from build123d import *

# Parameters (mm, degrees)
SKETCH_R        = 1.55
PAD_DEPTH       = 6.3
SKETCH001_W     = 3.4
SKETCH001_H     = 7.5
PAD001_DEPTH    = 6.3
SKETCH002_W     = 10
SKETCH002_H     = 19.4
PAD002_DEPTH    = 6
SKETCH003_R     = 1.65
POCKET_DEPTH    = 6.901
SKETCH004_R     = 1.65
POCKET001_DEPTH = 3.401
SKETCH005_R     = 2.2
POCKET002_DEPTH = 5
SKETCH006_W     = 5.6
SKETCH006_H     = 5.6
POCKET003_DEPTH = 2
SKETCH007_W     = 5.6
SKETCH007_H     = 5.6
POCKET004_DEPTH = 2
FILLET_R        = 4
CHAMFER_SIZE    = 5


with BuildPart() as part:
    # Sketch → Pad (new body)
    with BuildSketch(Plane.YZ):
        Polygon((-6.9, -4.5), (0, -4.5), (0, -19), (-15, -19), (-15, -11), (-6.9, -11), align=None)
        with Locations((-11, -15)):
            Circle(SKETCH_R, mode=Mode.SUBTRACT)
        with Locations((-4, -15)):
            Circle(SKETCH_R, mode=Mode.SUBTRACT)
    extrude(amount=PAD_DEPTH)

    # Sketch001 (on Face9 of Pad) → Pad001 (join)
    with BuildSketch(Plane(origin=(0, 0, 0), x_dir=(0, 1, 0), z_dir=(-1, 0, 0))):
        with Locations((-1.7, 8.25)):
            Rectangle(SKETCH001_W, SKETCH001_H)
    extrude(amount=PAD001_DEPTH)

    # Sketch002 (on Face11 of Pad001) → Pad002 (join)
    with BuildSketch(Plane(origin=(-6.3, 0, 0), x_dir=(0, 1, 0), z_dir=(-1, 0, 0))):
        with Locations((-5, 2.3)):
            Rectangle(SKETCH002_W, SKETCH002_H)
    extrude(amount=PAD002_DEPTH)

    # Sketch003 (on Face1 of Pad002) → Pocket (cut, through all)
    with BuildSketch(Plane(origin=(0, -6.9, 0), x_dir=(0, 0, -1), z_dir=(0, -1, 0))):
        with Locations((8.25, 3.15)):
            Circle(SKETCH003_R)
    extrude(amount=-POCKET_DEPTH, mode=Mode.SUBTRACT)

    # Sketch004 (on Face11 of Pocket) → Pocket001 (cut, through all)
    with BuildSketch(Plane(origin=(0, -3.4, 0), x_dir=(0, 0, -1), z_dir=(0, -1, 0))):
        with Locations((8.25, -3.15)):
            Circle(SKETCH004_R)
    extrude(amount=-POCKET001_DEPTH, mode=Mode.SUBTRACT)

    # Sketch005 (on Face18 of Pocket001) → Pocket002 (cut)
    with BuildSketch(Plane(origin=(0, -10, 0), x_dir=(0, 0, -1), z_dir=(0, -1, 0))):
        with Locations((-2.4, -9.3)):
            Circle(SKETCH005_R)
        with Locations((2.4, -9.3)):
            Circle(SKETCH005_R)
    extrude(amount=-POCKET002_DEPTH, mode=Mode.SUBTRACT)

    # Sketch006 (on Face3 of Pocket002) → Pocket003 (cut)
    with BuildSketch(Plane(origin=(0, 0, 0), x_dir=(0, 1, 0), z_dir=(-1, 0, 0))):
        with Locations((-4, 15)):
            Rectangle(SKETCH006_W, SKETCH006_H)
        with Locations((-11, 15)):
            Rectangle(SKETCH006_W, SKETCH006_H)
    extrude(amount=-POCKET003_DEPTH, mode=Mode.SUBTRACT)

    # Sketch007 (on Face11 of Pocket003) → Pocket004 (cut)
    with BuildSketch(Plane.ZX):
        with Locations((-8.25, 3.15)):
            Rectangle(SKETCH007_W, SKETCH007_H)
        with Locations((-8.25, -3.15)):
            Rectangle(SKETCH007_W, SKETCH007_H)
    extrude(amount=-POCKET004_DEPTH, mode=Mode.SUBTRACT)

    # Fillet
    fillet_edges = [part.edges().sort_by_distance(p)[0] for p in [
        (-12.3, -5, 7.4),
    ]]
    fillet(fillet_edges, radius=FILLET_R)

    # Chamfer
    chamfer_edges = [part.edges().sort_by_distance(p)[0] for p in [
        (-12.3, -5, -12),
    ]]
    chamfer(chamfer_edges, length=CHAMFER_SIZE)


solid = part.part
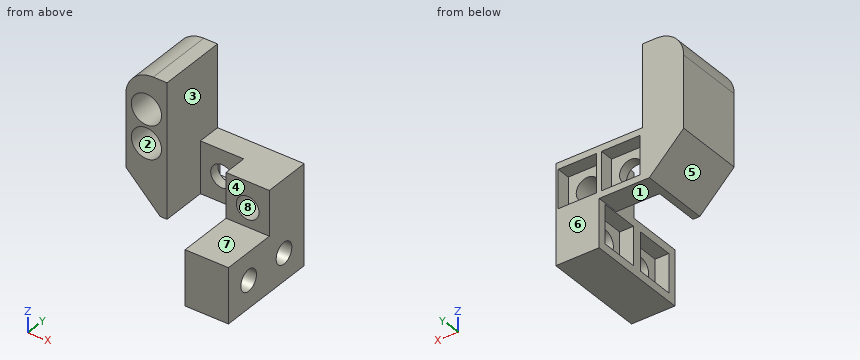
Source: CAD feature listing. Evaluate the final solid. Frame: model axes, mm. Face numbers are marked on the shaded views. A direction names the side the tool comes from. Coordinates: 2 decimals unless noted, no trailing zeros. Loops run counter-clockwise (first coordinate to the right, second up) from the corner with the lowest first, then second, coordinate; pieces in that order, holes last. Notation, with made-up numbers: M 57.5,47.25 L 89.5,47.25 A21 ccw 89.5,81.25 Z; hole C 58,54.5 d3. An arc over 180 degrees is marked long. Answer in a Markdown table with one row per item.
Q1. First-contact query: pin 1 (2 mm diameter, centred on x = -10, z = 3, fed in from -Y); pin 2 (1.6 mm diameter, centred on x = 1.5, y = -11.5, fed in from +Z); pin 3 (5 mm diameter, centred on x = -1, y = -2, fed in from +Z); pin 4 (3 mm diameter, centred on y = -11, z = -15, fed in from +X). Flat tips, straight axial feed; report the tip coordinate or a pass-through.
Answers below:
| item | result |
|---|---|
| pin 1 | stops at y = -5 |
| pin 2 | stops at z = -11 |
| pin 3 | stops at z = -4.5 |
| pin 4 | passes through |
Q2. Section A-A on y = -8.5. Return the cut outline in (x, z), plus the area to 3 significant figures.
Answers below:
| item | result |
|---|---|
| outline | M -12.3,-7 L -7.3,-12 L -6.3,-12 L -6.3,7.4 L -8.3,7.4 A4 ccw -12.3,3.4 Z; M 0,-19 L 6.3,-19 L 6.3,-11 L 0,-11 L 0,-12.2 L 2,-12.2 L 2,-17.8 L 0,-17.8 Z; hole C -9.3,-2.4 d4.4; hole C -9.3,2.4 d4.4 |
| area | 109 mm^2 |
Q3. Set-up query: the marked faces 1, 2, 3 and 4. Return all of +Z, -Z, +X, -X, +Y, -Y with unobstructed straight access to the full face (end or side cutting, diameter ignored); none if empty.
Answers below:
| item | result |
|---|---|
| face 1 | -Z, -X, +Y, -Y |
| face 2 | -Y |
| face 3 | +Z, -Y |
| face 4 | +Z, +X, -Y |
Q4. Section B-B on z = -15. Return the cut outline in (x, y).
Answers below:
| item | result |
|---|---|
| outline | M 0,-15 L 6.3,-15 L 6.3,-12.55 L 2,-12.55 L 2,-13.8 L 0,-13.8 Z; M 0,-8.2 L 2,-8.2 L 2,-9.45 L 6.3,-9.45 L 6.3,-5.55 L 2,-5.55 L 2,-6.8 L 0,-6.8 Z; M 0,-1.2 L 2,-1.2 L 2,-2.45 L 6.3,-2.45 L 6.3,0 L 0,0 Z |
Q5. Ray query, probe 1 along X at (y, z) = (-4.85, -8.25); probe 2 along X at (y, z) = (-3.05, -8.25); probe 3 along X at (y, z) = (-7.3, -2.4). Return the intervals inside material, ascending. Write a range as from..to.
Answers below:
| item | result |
|---|---|
| probe 1 | x = -11.05..-6.3, 0..1.5, 4.8..6.3 |
| probe 2 | x = -11.05..-4.8, -1.5..1.5, 4.8..6.3 |
| probe 3 | x = -12.3..-11.5, -7.1..-6.3 |
Q6. Section C-C on x = -3.15. Return the cut outline in (y, z), plus the area to 3 significant figures.
Answers below:
| item | result |
|---|---|
| outline | M -3.4,-12 L 0,-12 L 0,-11.05 L -2,-11.05 L -2,-9.9 L -3.4,-9.9 Z; M -3.4,-6.6 L -2,-6.6 L -2,-5.45 L 0,-5.45 L 0,-4.5 L -3.4,-4.5 Z |
| area | 9.68 mm^2 |
Q7. Draft query along Z for the marked faces 5, 6, 7 and 8. Return one class per face: pulls with the +Z half, pulls with the -Z half, needs draft (parallel to the pull), parting line crosses it, or undercut.
Answers below:
| item | result |
|---|---|
| face 5 | pulls with the -Z half |
| face 6 | needs draft |
| face 7 | pulls with the +Z half |
| face 8 | undercut |
Q8. Section D-D on y = -11. Return the cut outline in (x, z).
Answers below:
| item | result |
|---|---|
| outline | M 0,-19 L 6.3,-19 L 6.3,-16.55 L 2,-16.55 L 2,-17.8 L 0,-17.8 Z; M 0,-12.2 L 2,-12.2 L 2,-13.45 L 6.3,-13.45 L 6.3,-11 L 0,-11 Z |
